Here's how the part is built. I have some questions about the finished solid (model axes, mm). A direction names the side the tool comes from. Give positions to 0.01 mm unless a question says otherwise; leave off trailing zeros. Loops run counter-clockwise (first coordinate to the right, second up) from the corner with the lowest first, then second, coordinate; pieces in that order, holes last. Notation, with made-up numbers: (-6, 57) -> (29, 57) arc R21 ccw to (29, 76) -> close; hole circle Ø9 at (3.5, 51.25). An arc over 180 degrees is marked (long way). Answer in a Markdown table with one row per item. Add a question column.
Item 1: Which directions (+Z, -Z, +X, -X, +Y, -Y) give clear straight access to the entire face, cutting with the end or side of a thin tool? Please do faces 5 (the face through (56.3, 8, 88.9)), 6 (the face through (-28, 10, 78)), 7 (the face through (-1.63, 1.48, 34.26)).
Item 2: If we section it at A-A (y = 5.75): Write out the boundary of the cut face in (x, z), then the cut area to 3 significant figures.
Item 3: For P1, Ø6, axis at x = 33.5, z = 104, coming from the -Y side, with a flat end and sliding along its axis, tell me the tip position at first contact or that it passes through.
Item 4: We'd pull the mould along X, two halves only. Please class faces 1 (the face through (-82.637, 5, 82)), 2 (the face through (89.38, 5.07, -20.77)), 3 (the face through (117.363, 5, 82)), 4 (the face through (17.13, 8.125, 81.124)): released by +X, released by -X, zero draft, split by the parting line, or undercut.
Item 5: If I drill on line 1 (Z direction, x = 102.5, y = 2.75); line 2 (Z direction, x = -68, y = 9.75) (3 decimals); line 3 (Z direction, x = -25, y = 1), over which ranges is the centre line in solid material (lowest first)?
```python
from build123d import *

# Parameters (mm, degrees)
SKETCH1_W           = 200
SKETCH1_H           = 255
BOSS_EXTRUDE1_DEPTH = 10
SKETCH2_R           = 49.592553134
CUT_EXTRUDE1_DEPTH  = 3
SKETCH3_R           = 9
CUT_EXTRUDE2_DEPTH  = 69
SKETCH4_R           = 42.638858135
SKETCH4_R_2         = 37.540647577
CUT_EXTRUDE3_DEPTH  = 2
CUT_EXTRUDE3_DRAFT  = -45
FILLET1_R           = 4
FILLET2_R           = 4
SKETCH5_R           = 2.952313346
CUT_EXTRUDE4_DEPTH  = 2
CUT_EXTRUDE4_DRAFT  = -45


with BuildPart() as part:
    # Sketch1 → Boss-Extrude1 (new body)
    with BuildSketch(Plane(origin=(0, 0, 0), x_dir=(1, 0, 0), z_dir=(0, 1, 0))):
        with Locations((17.363344051, -80.072347267)):
            Rectangle(SKETCH1_W, SKETCH1_H)
    extrude(amount=BOSS_EXTRUDE1_DEPTH)

    # Sketch2 → Cut-Extrude1 (cut)
    with BuildSketch(Plane(origin=(0, 0, 0), x_dir=(-1, 0, 0), z_dir=(0, -1, 0))):
        with Locations(Location((-17.363344051, -80.072347267, 0), (0, 0, 90))):
            Circle(SKETCH2_R)
    extrude(amount=-CUT_EXTRUDE1_DEPTH, mode=Mode.SUBTRACT)

    # Sketch3 → Cut-Extrude2 (cut)
    with BuildSketch(Plane(origin=(0, 10, 0), x_dir=(1, 0, 0), z_dir=(0, 1, 0))):
        with Locations(Location((97.363344051, -185.072347267, 0), (0, 0, 270))):
            Circle(SKETCH3_R)
        with Locations(Location((-62.636655949, 24.927652733, 0), (0, 0, 270))):
            Circle(SKETCH3_R)
        with Locations(Location((-62.636655949, -185.072347267, 0), (0, 0, 270))):
            Circle(SKETCH3_R)
        with Locations(Location((97.363344051, 24.927652733, 0), (0, 0, 270))):
            Circle(SKETCH3_R)
    extrude(amount=-CUT_EXTRUDE2_DEPTH, mode=Mode.SUBTRACT)


with BuildPart() as cut_extrude3_tool:
    # Sketch4 → Cut-Extrude3 (with draft: the straight prism first)
    with BuildSketch(Plane(origin=(0, 10, 0), x_dir=(1, 0, 0), z_dir=(0, 1, 0))):
        with Locations((17.363344051, -80.072347267)):
            Circle(SKETCH4_R)
        with Locations((17.363344051, -80.072347267)):
            Circle(SKETCH4_R_2, mode=Mode.SUBTRACT)
    extrude(amount=-CUT_EXTRUDE3_DEPTH)
    # Cut-Extrude3: the draft: its side faces are tilted about the plane it starts from
    cut_extrude3_sides = [cut_extrude3_tool.faces().sort_by_distance(p)[0] for p in [
        (-25.275514084, 9, 80.072347267),
        (-20.177303525, 9, 80.072347267),
    ]]
    draft(cut_extrude3_sides, Plane(origin=(0, 10, 0), x_dir=(1, 0, 0), z_dir=(0, 1, 0)), CUT_EXTRUDE3_DRAFT)


with BuildPart() as part_1:
    add(part.part)

    # Cut-Extrude3: cut by cut_extrude3_tool
    add(cut_extrude3_tool.part, mode=Mode.SUBTRACT)

    # Fillet1
    fillet1_edges = [part_1.edges().sort_by_distance(p)[0] for p in [
        (-25.275514084, 10, 80.072347267),
    ]]
    fillet(fillet1_edges, radius=FILLET1_R)

    # Fillet2
    fillet2_edges = [part_1.edges().sort_by_distance(p)[0] for p in [
        (-20.177303525, 10, 80.072347267),
    ]]
    fillet(fillet2_edges, radius=FILLET2_R)


with BuildPart() as cut_extrude4_tool:
    # Sketch5 → Cut-Extrude4 (with draft: the straight prism first)
    with BuildSketch(Plane(origin=(0, 10, 0), x_dir=(1, 0, 0), z_dir=(0, 1, 0))):
        with Locations((17.363344051, -80.072347267)):
            Circle(SKETCH5_R)
    extrude(amount=-CUT_EXTRUDE4_DEPTH)
    # Cut-Extrude4: the draft: its side faces are tilted about the plane it starts from
    cut_extrude4_sides = [cut_extrude4_tool.faces().sort_by_distance(p)[0] for p in [
        (14.411030705, 9, 80.072347267),
    ]]
    draft(cut_extrude4_sides, Plane(origin=(0, 10, 0), x_dir=(1, 0, 0), z_dir=(0, 1, 0)), CUT_EXTRUDE4_DRAFT)


with BuildPart() as part_2:
    add(part_1.part)

    # Cut-Extrude4: cut by cut_extrude4_tool
    add(cut_extrude4_tool.part, mode=Mode.SUBTRACT)


solid = part_2.part
```
Recorded:
| question | item | result |
|---|---|---|
| 1 | face 5 | +Y |
| 1 | face 6 | +Z, -Z, +X, -X, +Y |
| 1 | face 7 | -Y |
| 2 | outline | (-82.64, -47.43) -> (117.36, -47.43) -> (117.36, 207.57) -> (-82.64, 207.57) -> close; hole circle Ø18 at (-62.64, -24.93); hole circle Ø18 at (-62.64, 185.07); hole circle Ø18 at (97.36, -24.93); hole circle Ø18 at (97.36, 185.07) |
| 2 | area | 50,000 mm^2 |
| 3 | P1 | stops at y = 3 |
| 4 | face 1 | released by -X |
| 4 | face 2 | undercut |
| 4 | face 3 | released by +X |
| 4 | face 4 | undercut |
| 5 | line 1 | z = -47.43 to -32.32, -17.54 to 177.68, 192.46 to 207.57 |
| 5 | line 2 | z = -47.428 to -32.155, -17.7 to 177.845, 192.3 to 207.572 |
| 5 | line 3 | z = -47.43 to 54.29, 105.86 to 207.57 |
